```python
from build123d import *

# Parameters (mm, degrees)
BASE_EXTRUDE_DEPTH = 55.5752
SKETCH2_R          = 31.75
CUT_EXTRUDE1_DEPTH = 96.446823878


with BuildPart() as part:
    # Sketch1 → Base-Extrude (new body)
    with BuildSketch(Plane(origin=(0, 0, 0), x_dir=(1, 0, 0), z_dir=(0, 1, 0))):
        Polygon((58.65878735, 0), (29.329393675, 50.8), (-29.329393675, 50.8), (-58.65878735, 0), (-29.329393675, -50.8), (29.329393675, -50.8), align=None)
    extrude(amount=BASE_EXTRUDE_DEPTH)

    # Sketch2 → Cut-Extrude1 (cut, through all)
    with BuildSketch(Plane(origin=(0, 0, 0), x_dir=(-1, 0, 0), z_dir=(0, -1, 0))):
        with Locations(Location((0, 0, 0), (0, 0, 90))):
            Circle(SKETCH2_R)
    extrude(amount=-CUT_EXTRUDE1_DEPTH, mode=Mode.SUBTRACT)

    # Sketch10 → Cut-Revolve3 (revolve, cut)
    with BuildSketch(Plane.XY, mode=Mode.PRIVATE) as cut_revolve3_sk:
        with BuildLine():
            Line((0, 56.8452), (59.9186, 56.8452))
            Line((59.9186, 56.8452), (59.9186, -1.27))
            Line((59.9186, -1.27), (0, -1.27))
            Line((0, -1.27), (0, 0))
            Line((0, 0), (50.81018735, 0))
            Line((50.81018735, 0), (58.65878735, 3.659862286))
            Line((58.65878735, 3.659862286), (58.65878735, 42.639587275))
            Line((58.65878735, 42.639587275), (50.8, 46.3042))
            ThreePointArc((50.8, 46.3042), (48.084586968, 52.859786968), (41.529, 55.5752))
            Line((41.529, 55.5752), (0, 55.5752))
            Line((0, 55.5752), (0, 56.8452))
        make_face()
    revolve(cut_revolve3_sk.sketch.rotate(Axis((0, 55.5752, 0), (0, -1, 0)), 90), axis=Axis((0, 55.5752, 0), (0, -1, 0)), mode=Mode.SUBTRACT)


solid = part.part
```
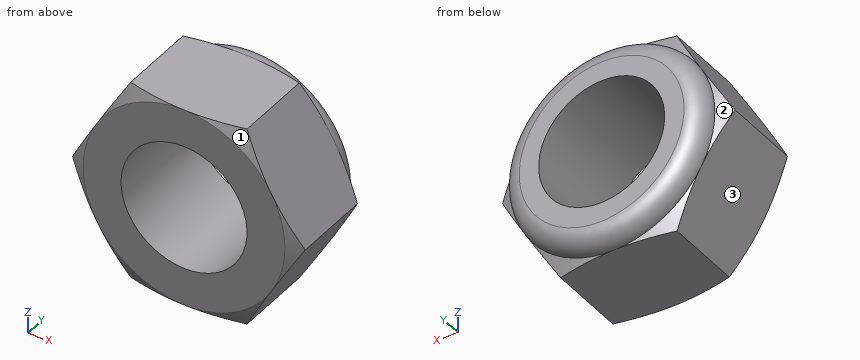
Geometry check sheet. Reference: the model listing, model coordinates, mm. Face numbers are marked on the shaded views. Round coordinates to 2 decimals unless told otherwise and drop trailing zeros. Loops run counter-clockwise (first coordinate to the right, second up) from the corner with the lowest first, then second, coordinate; pieces in that order, holes last. Notation, with made-up numbers: M 42,-7.75 L 80,-7.75 A7 cw 80,1.25 Z; hole C -29,67 d9. An arc over 180 degrees is marked long. Return JSON: item names as keys, results as strings. Group by question number.
(1) Section check A-A, the plane y = 22. Enter the section's corners in (x, z), and give its area (3 significant figures).
(2) Go/stop test with flat-tipped pins: pin 1 (1.5 mm diameter, centred on y = 13, z = -37.5, fed in from +X); pin 2 (4 mm diameter, centred on y = 48, z = 4, fed in from -X); pin 3 (2 mm diameter, centred on y = 11.5, z = -27, fed in from -X). Record where each tip stops, or that it passes through.
(3) Scan lines: line 1 along X through (y, z) = (22, 0); line 2 along Y through (x, z) = (36.5, 20); line 3 along X through (y, z) = (32, -15). Record each from-to range of solid material in increasing order. Write a range as [from, to].
(4) Mould release check, pull along Y, two halves, no side actions. Record for the marked faces 1, 2 and 3: pulls with the +Y half, pulls with the -Y half, needs draft (parallel to the pull), parting line crosses it, or undercut.
Data:
{
 "1": {"outline": "M -58.66,0 L -29.33,-50.8 L 29.33,-50.8 L 58.66,0 L 29.33,50.8 L -29.33,50.8 Z; hole C 0,0 d63.5", "area": "5,770 mm²"},
 "2": {"pin 1": "x = 37.44", "pin 2": "x = -51.3", "pin 3": "x = -43.65"},
 "3": {"line 1": "[-58.66, -31.75], [31.75, 58.66]", "line 2": "[0, 55.57]", "line 3": "[-50, -27.98], [27.98, 50]"},
 "4": {"face 1": "pulls with the -Y half", "face 2": "pulls with the +Y half", "face 3": "needs draft"}
}
